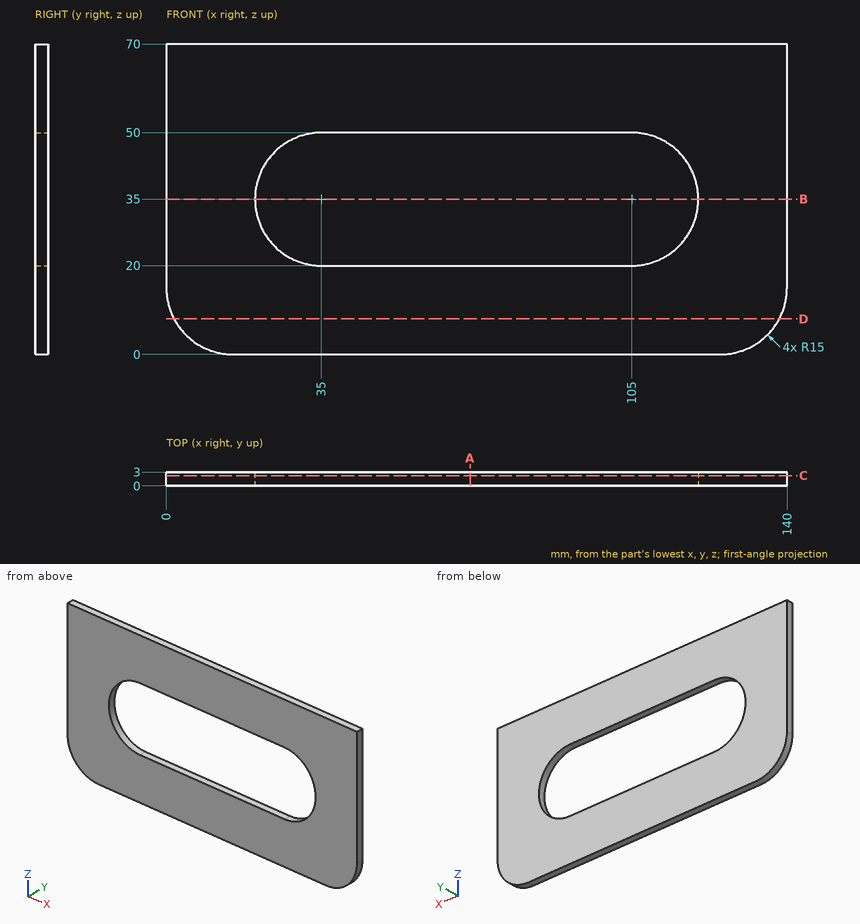
Print and shaded views of the part. All mm, measured from the part's lowest x, y and z. Give positions to 0.01 mm unless a question says otherwise; leave off trailing zeros. Loops run counter-clockwise (first coordinate to the right, second up) from the corner with the lowest first, then second, coordinate; pieces in that order, holes last. Notation, with made-up numbers: (-6, 30.5) -> (7, 30.5) arc R28 cw to (7, 56.5) -> close; hole circle Ø5 at (33, 73). An arc over 180 degrees is marked (long way). Use a Markdown table: item, result.
1. Slice it at B-B (z = 35). List the corners of the cut face in (x, y), plus the area to 3 significant figures.
Check result:
| item | result |
|---|---|
| outline | (0, 0) -> (20, 0) -> (20, 3) -> (0, 3) -> close; (120, 0) -> (140, 0) -> (140, 3) -> (120, 3) -> close |
| area | 120 mm^2 |
2. Wall check: L1, parallel to Z at x = 84.5, y = 0.75; L2, parallel to X at y = 1.6, z = 48.5; L3, parallel to X at y = 2, z = 32. Give the ranges that are in metal, low to high. Write a range as [from, to].
Check result:
| item | result |
|---|---|
| L1 | z = [0, 20], [50, 70] |
| L2 | x = [0, 28.46], [111.54, 140] |
| L3 | x = [0, 20.3], [119.7, 140] |
3. Slice it at D-D (z = 8). List the corners of the cut face in (x, y).
Check result:
| item | result |
|---|---|
| outline | (1.73, 0) -> (138.27, 0) -> (138.27, 3) -> (1.73, 3) -> close |
4. Slice it at A-A (x = 68.5). List the corners of the cut face in (y, z).
Check result:
| item | result |
|---|---|
| outline | (0, 0) -> (3, 0) -> (3, 20) -> (0, 20) -> close; (0, 50) -> (3, 50) -> (3, 70) -> (0, 70) -> close |
5. Flat gauge pin, fed straight in: pin 1 (6 mm diameter, centred on x = 18.5, z = 32.5, fed in from -Y). Where does the tip first touch, or does it go through?
Check result:
| item | result |
|---|---|
| pin 1 | stops at y = 0 |
6. Slice it at C-C (y = 2.25). List the corners of the cut face in (x, z), plus the area to 3 significant figures.
Check result:
| item | result |
|---|---|
| outline | (0, 15) arc R15 ccw to (15, 0) -> (125, 0) arc R15 ccw to (140, 15) -> (140, 70) -> (0, 70) -> close; hole (35, 20) -> (105, 20) arc R15 ccw to (105, 50) -> (35, 50) arc R15 ccw to start |
| area | 6,900 mm^2 |
